Here's how the part is built. I have some questions about the finished solid (model axes, mm). A direction names the side the tool comes from. Round coordinates to 2 decimals unless told otherwise and drop trailing zeros. Loops run counter-clockwise (first coordinate to the right, second up) from the corner with the lowest first, then second, coordinate; pieces in that order, holes last. Notation, with made-up numbers: M -11.75,36 L 18.25,36 A21 ccw 18.25,56 Z; hole C -12.5,-3.75 d5. An arc over 180 degrees is marked long. Use a Markdown table: item, result.
Autodesk Inventor part; units mm, degrees
ref_plane "YZ Plane" through (0, 0, 0) normal (1, 0, 0) x (0, 1, 0)
ref_plane "XZ Plane" through (0, 0, 0) normal (0, 1, 0) x (-1, 0, 0)
ref_plane "XY Plane" through (0, 0, 0) normal (0, 0, 1) x (1, 0, 0)
sketch "Sketch1" plane through (0, 0, 0) normal (0, 1, 0) x (-1, 0, 0)
  line L0 (0, 0) -> (37, 0)
  line L1 (37, 0) -> (37, -20)
  line L2 (37, -20) -> (0, -20)
  line L3 (0, -20) -> (0, 0)
  dimension "d0" = 37
  dimension "d1" = 20
extrude "Extrusion1" add sketch "Sketch1" along normal blind 6
sketch "Sketch2" plane through (0, 6, 0) normal (0, 1, 0) x (1, 0, 0)
  circle A0 centre (-10, 5) radius 2.5
  circle A1 centre (-10, 15) radius 2.5
  line L0 (0, 0) -> (0, 20)
  line L1 (0, 20) -> (-37, 20)
  line L2 (-37, 0) -> (0, 0)
  dimension "d4" = 5
  dimension "d5" = 5
  dimension "d6" = 10
  dimension "d7" = 10
  dimension "d8" = 5
  dimension "d9" = 5
extrude "Extrusion2" cut sketch "Sketch2" against normal blind 8
sketch "Sketch3" plane through (-37, 0, -20) normal (-1, 0, 0) x (0, 0, 1)
  circle A0 centre (5.25, 3) radius 1
  circle A1 centre (14.75, 3) radius 1
  line L0 (0, 0) -> (20, 0)
  line L1 (0, 0) -> (0, 6)
  dimension "d12" = 2
  dimension "d13" = 2
  dimension "d14" = 9.5
  dimension "d15" = 3
  dimension "d16" = 3
  dimension "d17" = 5.25
extrude "Extrusion3" cut sketch "Sketch3" against normal blind 20
thread "Thread1"
thread "Thread2"
properties part number "Endstop_holer_X"
1. Imagine slicing it at B-B, the plane y = 3. Write out the boundary of the cut face in (x, z).
Answer sheet:
| item | result |
|---|---|
| outline | M -37,-20 L 0,-20 L 0,0 L -37,0 L -37,-4.25 L -17,-4.25 L -17,-6.25 L -37,-6.25 L -37,-13.75 L -17,-13.75 L -17,-15.75 L -37,-15.75 Z; hole C -10,-15 d5; hole C -10,-5 d5 |
2. For pin 1 Ø3 at (x, z) = (-10, -15) entering from +Y; pin 2 Ø1.8 at (y, z) = (3, -14.75) entering from -X, each with a flat end and sliding along its axis, tell me the tip position at first contact or that it passes through.
Answer sheet:
| item | result |
|---|---|
| pin 1 | through |
| pin 2 | x = -17 |
3. I need wall thicknesses on probe 1 along Z at (x, y) = (-10, 1.65); probe 2 along Z at (x, y) = (-31, 3.5); probe 3 along X at (y, z) = (3.3, -15). Which ranges of each line are inside material? Lowest first, please. Write a range as from..to.
Answer sheet:
| item | result |
|---|---|
| probe 1 | -20..-17.5, -12.5..-7.5, -2.5..0 |
| probe 2 | -20..-15.62, -13.88..-6.12, -4.38..0 |
| probe 3 | -17..-12.5, -7.5..0 |
4. We'd pull the mould along X, two halves only. Please class faces 3 (the face through (-12, 3, -13.5)), 4 (the face through (-17, 3, -5)), 5 (the face through (-11.84, 3.04, -6.69)), 6 (the face through (-18, 3, 0)): +X half, -X half, draft (parallel to the pull), parting line (faces both ways), or undercut.
Answer sheet:
| item | result |
|---|---|
| face 3 | undercut |
| face 4 | -X half |
| face 5 | undercut |
| face 6 | draft |
5. Imagine slicing it at D-D, the plane z = -14.25. Write out the boundary of the cut face in (x, y), then the cut area to 3 significant figures.
Answer sheet:
| item | result |
|---|---|
| outline | M -37,0 L -12.38,0 L -12.38,6 L -37,6 L -37,3.87 L -17,3.87 L -17,2.13 L -37,2.13 Z; M -7.62,0 L 0,0 L 0,6 L -7.62,6 Z |
| area | 159 mm2 |
6. Imagine slicing it at A-A, the plane x = -12. Write out the boundary of the cut face in (y, z), then the cut area to 3 significant figures.
Answer sheet:
| item | result |
|---|---|
| outline | M 0,-20 L 6,-20 L 6,-16.5 L 0,-16.5 Z; M 0,-13.5 L 6,-13.5 L 6,-6.5 L 0,-6.5 Z; M 0,-3.5 L 6,-3.5 L 6,0 L 0,0 Z |
| area | 84.0 mm2 |
7. Which directions (+Z, -Z, +X, -X, +Y, -Y) give clear straight access to the entire face, cutting with the end or side of a thin tool? Please do faces 1 (the face through (-37, 3, -10)), 2 (the face through (-27.14, 3.676, -5.987)).
Answer sheet:
| item | result |
|---|---|
| face 1 | +Z, -Z, -X, +Y, -Y |
| face 2 | -X |
8. Imagine slicing it at C-C, the plane x = -20. Write out the boundary of the cut face in (y, z).
Answer sheet:
| item | result |
|---|---|
| outline | M 0,-20 L 6,-20 L 6,0 L 0,0 Z; hole C 3,-14.75 d2; hole C 3,-5.25 d2 |
